For this review, take the finished solid that the model builds, in its own axes (mm). Give positions to 0.01 mm unless a question says otherwise; leave off trailing zeros. Write each loop counter-clockwise with the first axis right and the second up, starting at its lowest first coordinate (ties: lowest second). Pieces come first, ordered by that corner, then holes.
Q1. For line 1 (X direction, y = 5.5, z = 50.8); line 2 (Z direction, x = 25.4, y = 11.5); line 3 (X direction, y = 12, z = 1), list the stretches that pass through material, from the lowest coordinate up.
Q2. We need section C-C (x = -50.8). Write out the cut boundary in (y, z).
Q3. We need section B-B (y = 13.25). Give the number of separate pieces and of enclosed holes in the cut face, then the cut area to 3 significant figures.
Q4. We need section A-A (z = -50.8). Write out the cut boundary in (x, y).
Q5. Mouldability with a two-part tool opening along X and no side actions: class faces 1 (the cylindrical face through (0.33, 9.39, -53.33)), 2 (the flat face through (57.15, 9, 1)), 3 (the flat face through (-1, 9, -76.2)) as released by +X, released by -X, zero draft, split by the parting line, or undercut.
```python
from build123d import *

# Parameters (mm, degrees)
SKETCH1_W               = 114.3
SKETCH1_H               = 152.4
BOSS_EXTRUDE1_DEPTH     = 19.05
F_1_4_20_TAPPED_HOLE1_D = 5.1054
LPATTERN1_COUNT         = 3
LPATTERN1_PITCH         = 25.4
LPATTERN1_COL_COUNT     = 3
LPATTERN1_COL_PITCH     = 25.4
LPATTERN2_COUNT         = 3
LPATTERN2_PITCH         = 25.4
LPATTERN2_COPY_1_D      = 5.1054
LPATTERN2_COPY_2_D      = 5.1054
LPATTERN2_COPY_3_D      = 5.1054
LPATTERN2_COPY_4_D      = 5.1054
LPATTERN2_COPY_5_D      = 5.1054
LPATTERN2_COPY_6_D      = 5.1054
LPATTERN2_COPY_7_D      = 5.1054
LPATTERN2_COPY_8_D      = 5.1054
LPATTERN2_COL_COUNT     = 3
LPATTERN2_COL_PITCH     = 25.4
LPATTERN2_COL_COPY_1_D  = 5.1054
LPATTERN2_COL_COPY_2_D  = 5.1054
LPATTERN2_COL_COPY_3_D  = 5.1054
LPATTERN2_COL_COPY_4_D  = 5.1054
LPATTERN2_COL_COPY_5_D  = 5.1054
LPATTERN2_COL_COPY_6_D  = 5.1054
LPATTERN2_COL_COPY_7_D  = 5.1054
LPATTERN2_COL_COPY_8_D  = 5.1054


with BuildPart() as part:
    # Sketch1 → Boss-Extrude1 (new body)
    with BuildSketch(Plane(origin=(0, 0, 0), x_dir=(1, 0, 0), z_dir=(0, 1, 0))):
        Rectangle(SKETCH1_W, SKETCH1_H)
    extrude(amount=BOSS_EXTRUDE1_DEPTH)

    # 1/4-20 Tapped Hole1 (through all)
    with Locations(Plane(origin=(0, 19.05, 0), x_dir=(1, 0, 0), z_dir=(0, 1, 0))):
        with Locations((0, 0)):
            f_1_4_20_tapped_hole1 = Hole(F_1_4_20_TAPPED_HOLE1_D / 2)

    # LPattern1: 1/4-20 Tapped Hole1 ×3
    with Locations(*[(0, 0, i * LPATTERN1_PITCH) for i in range(1, LPATTERN1_COUNT)]):
        add(f_1_4_20_tapped_hole1, mode=Mode.SUBTRACT)

    # LPattern1 col: 1/4-20 Tapped Hole1 ×3
    with Locations(*[(0, 0, -i * LPATTERN1_COL_PITCH) for i in range(1, LPATTERN1_COL_COUNT)]):
        add(f_1_4_20_tapped_hole1, mode=Mode.SUBTRACT)

    # LPattern2: 1/4-20 Tapped Hole1 ×3
    with Locations(*[(i * LPATTERN2_PITCH, 0, 0) for i in range(1, LPATTERN2_COUNT)]):
        add(f_1_4_20_tapped_hole1, mode=Mode.SUBTRACT)

    # LPattern2 copy 1 (through all)
    with Locations(Plane(origin=(25.4, 19.05, 25.4), x_dir=(1, 0, 0), z_dir=(0, 1, 0))):
        with Locations((0, 0)):
            Hole(LPATTERN2_COPY_1_D / 2)

    # LPattern2 copy 2 (through all)
    with Locations(Plane(origin=(50.8, 19.05, 25.4), x_dir=(1, 0, 0), z_dir=(0, 1, 0))):
        with Locations((0, 0)):
            Hole(LPATTERN2_COPY_2_D / 2)

    # LPattern2 copy 3 (through all)
    with Locations(Plane(origin=(25.4, 19.05, 50.8), x_dir=(1, 0, 0), z_dir=(0, 1, 0))):
        with Locations((0, 0)):
            Hole(LPATTERN2_COPY_3_D / 2)

    # LPattern2 copy 4 (through all)
    with Locations(Plane(origin=(50.8, 19.05, 50.8), x_dir=(1, 0, 0), z_dir=(0, 1, 0))):
        with Locations((0, 0)):
            Hole(LPATTERN2_COPY_4_D / 2)

    # LPattern2 copy 5 (through all)
    with Locations(Plane(origin=(25.4, 19.05, -25.4), x_dir=(1, 0, 0), z_dir=(0, 1, 0))):
        with Locations((0, 0)):
            Hole(LPATTERN2_COPY_5_D / 2)

    # LPattern2 copy 6 (through all)
    with Locations(Plane(origin=(50.8, 19.05, -25.4), x_dir=(1, 0, 0), z_dir=(0, 1, 0))):
        with Locations((0, 0)):
            Hole(LPATTERN2_COPY_6_D / 2)

    # LPattern2 copy 7 (through all)
    with Locations(Plane(origin=(25.4, 19.05, -50.8), x_dir=(1, 0, 0), z_dir=(0, 1, 0))):
        with Locations((0, 0)):
            Hole(LPATTERN2_COPY_7_D / 2)

    # LPattern2 copy 8 (through all)
    with Locations(Plane(origin=(50.8, 19.05, -50.8), x_dir=(1, 0, 0), z_dir=(0, 1, 0))):
        with Locations((0, 0)):
            Hole(LPATTERN2_COPY_8_D / 2)

    # LPattern2 col: 1/4-20 Tapped Hole1 ×3
    with Locations(*[(-i * LPATTERN2_COL_PITCH, 0, 0) for i in range(1, LPATTERN2_COL_COUNT)]):
        add(f_1_4_20_tapped_hole1, mode=Mode.SUBTRACT)

    # LPattern2 col copy 1 (through all)
    with Locations(Plane(origin=(-25.4, 19.05, 25.4), x_dir=(1, 0, 0), z_dir=(0, 1, 0))):
        with Locations((0, 0)):
            Hole(LPATTERN2_COL_COPY_1_D / 2)

    # LPattern2 col copy 2 (through all)
    with Locations(Plane(origin=(-50.8, 19.05, 25.4), x_dir=(1, 0, 0), z_dir=(0, 1, 0))):
        with Locations((0, 0)):
            Hole(LPATTERN2_COL_COPY_2_D / 2)

    # LPattern2 col copy 3 (through all)
    with Locations(Plane(origin=(-25.4, 19.05, 50.8), x_dir=(1, 0, 0), z_dir=(0, 1, 0))):
        with Locations((0, 0)):
            Hole(LPATTERN2_COL_COPY_3_D / 2)

    # LPattern2 col copy 4 (through all)
    with Locations(Plane(origin=(-50.8, 19.05, 50.8), x_dir=(1, 0, 0), z_dir=(0, 1, 0))):
        with Locations((0, 0)):
            Hole(LPATTERN2_COL_COPY_4_D / 2)

    # LPattern2 col copy 5 (through all)
    with Locations(Plane(origin=(-25.4, 19.05, -25.4), x_dir=(1, 0, 0), z_dir=(0, 1, 0))):
        with Locations((0, 0)):
            Hole(LPATTERN2_COL_COPY_5_D / 2)

    # LPattern2 col copy 6 (through all)
    with Locations(Plane(origin=(-50.8, 19.05, -25.4), x_dir=(1, 0, 0), z_dir=(0, 1, 0))):
        with Locations((0, 0)):
            Hole(LPATTERN2_COL_COPY_6_D / 2)

    # LPattern2 col copy 7 (through all)
    with Locations(Plane(origin=(-25.4, 19.05, -50.8), x_dir=(1, 0, 0), z_dir=(0, 1, 0))):
        with Locations((0, 0)):
            Hole(LPATTERN2_COL_COPY_7_D / 2)

    # LPattern2 col copy 8 (through all)
    with Locations(Plane(origin=(-50.8, 19.05, -50.8), x_dir=(1, 0, 0), z_dir=(0, 1, 0))):
        with Locations((0, 0)):
            Hole(LPATTERN2_COL_COPY_8_D / 2)


solid = part.part
```
Computed:
1. line 1: x = -57.15 to -53.35, -48.25 to -27.95, -22.85 to -2.55, 2.55 to 22.85, 27.95 to 48.25, 53.35 to 57.15
1. line 2: z = -76.2 to -53.35, -48.25 to -27.95, -22.85 to -2.55, 2.55 to 22.85, 27.95 to 48.25, 53.35 to 76.2
1. line 3: x = -57.15 to -53.15, -48.45 to -27.75, -23.05 to -2.35, 2.35 to 23.05, 27.75 to 48.45, 53.15 to 57.15
2. outline: (0, -76.2) - (19.05, -76.2) - (19.05, -53.35) - (0, -53.35) - close; (0, -48.25) - (19.05, -48.25) - (19.05, -27.95) - (0, -27.95) - close; (0, -22.85) - (19.05, -22.85) - (19.05, -2.55) - (0, -2.55) - close; (0, 2.55) - (19.05, 2.55) - (19.05, 22.85) - (0, 22.85) - close; (0, 27.95) - (19.05, 27.95) - (19.05, 48.25) - (0, 48.25) - close; (0, 53.35) - (19.05, 53.35) - (19.05, 76.2) - (0, 76.2) - close
3. separate pieces: 1
3. enclosed holes: 25
3. area: 16,900 mm2
4. outline: (-57.15, 0) - (-53.35, 0) - (-53.35, 19.05) - (-57.15, 19.05) - close; (-48.25, 0) - (-27.95, 0) - (-27.95, 19.05) - (-48.25, 19.05) - close; (-22.85, 0) - (-2.55, 0) - (-2.55, 19.05) - (-22.85, 19.05) - close; (2.55, 0) - (22.85, 0) - (22.85, 19.05) - (2.55, 19.05) - close; (27.95, 0) - (48.25, 0) - (48.25, 19.05) - (27.95, 19.05) - close; (53.35, 0) - (57.15, 0) - (57.15, 19.05) - (53.35, 19.05) - close
5. face 1: undercut
5. face 2: released by +X
5. face 3: zero draft
